```python
from build123d import *

# Parameters (mm, degrees)
EXTRUDE_1_DEPTH            = 7.5
EXTRUDE_1_DEPTH_BACK       = 7.5
SKETCH_3_W                 = 10
SKETCH_3_H                 = 21
CUT_EXTRUDE_1_DEPTH        = 29.062430401
SKETCH_4_W                 = 3
SKETCH_4_H                 = 3
EXTRUDE_2_DEPTH            = 1
EXTRUDE_3_DEPTH            = 2
EXTRUDE_3_DEPTH_BACK       = 2
CUT_EXTRUDE_2_REACH        = 27.53
SKETCH_7_W                 = 3
SKETCH_7_H                 = 3
EXTRUDE_4_DEPTH            = 1
EXTRUDE_START              = -4
EXTRUDE_5_DEPTH            = 5
CUT_EXTRUDE_3_REACH        = 28.373
SKETCH_10_R                = 1.9
EXTRUDE_6_DEPTH            = 1.5
EXTRUDE_START_2            = 1.5
SKETCH_11_R                = 1.9
EXTRUDE_7_DEPTH            = 1.5
EXTRUDE_8_DEPTH            = 0.5
EXTRUDE_8_DEPTH_BACK       = 0.5
SKETCH_13_W                = 12
SKETCH_13_H                = 1.5
EXTRUDE_9_DEPTH            = 1
CHAMFER_1_SIZE             = 1
CHAMFER_1_OF_MIRROR_2_SIZE = 1
FILLET_1_R                 = 0.1
FILLET_2_R                 = 0.2
FILLET_3_R                 = 0.2
FILLET_4_R                 = 0.1


with BuildPart() as part:
    # Sketch 1 → Extrude 1 (new, two sides: drawn at the far end of the back side and taken through both)
    with BuildSketch(Plane.XY.offset(-EXTRUDE_1_DEPTH_BACK)):
        with BuildLine():
            Line((-7.5, 0), (7.5, 0))
            Line((7.5, 0), (7.5, 15))
            ThreePointArc((7.5, 15), (0, 22.5), (-7.5, 15))
            Line((-7.5, 15), (-7.5, 0))
        make_face()
    extrude(amount=EXTRUDE_1_DEPTH + EXTRUDE_1_DEPTH_BACK)

    # Sketch 3 → Cut-Extrude 1 (cut, through all)
    with BuildSketch(Plane.ZY.offset(7.5)):
        with Locations((0, 12)):
            Rectangle(SKETCH_3_W, SKETCH_3_H)
    extrude(amount=-CUT_EXTRUDE_1_DEPTH, mode=Mode.SUBTRACT)

    # Sketch 4 → Extrude 2 (add)
    with BuildSketch(Plane(origin=(0, 0, 0), x_dir=(-1, 0, 0), z_dir=(0, -1, 0))):
        Rectangle(SKETCH_4_W, SKETCH_4_H)
    extrude(amount=EXTRUDE_2_DEPTH)

    # Sketch 5 → Extrude 3 (add, two sides: drawn at the far end of the back side and taken through both)
    with BuildSketch(Plane.XY.offset(-EXTRUDE_3_DEPTH_BACK)):
        with BuildLine():
            Line((-1.95, -2.5), (1.95, -2.5))
            Line((1.95, -2.5), (1.95, -1.555590279))
            ThreePointArc((1.95, -1.555590279), (1.780042303, -1.088161527), (1.5, -0.677124344))
            Line((1.5, -0.677124344), (-1.5, -0.677124344))
            ThreePointArc((-1.5, -0.677124344), (-1.780042303, -1.088161527), (-1.95, -1.555590279))
            Line((-1.95, -1.555590279), (-1.95, -2.5))
        make_face()
    extrude(amount=EXTRUDE_3_DEPTH + EXTRUDE_3_DEPTH_BACK)

    # Sketch 6 → Cut-Extrude 2 (cut, up to next)
    with BuildSketch(Plane.ZY.offset(1.95), mode=Mode.PRIVATE) as cut_extrude_2_sk1:
        with BuildLine():
            Line((-1.95, -2.5), (-1.95, -1.555590279))
            ThreePointArc((-1.95, -1.555590279), (-1.780042303, -1.088161527), (-1.5, -0.677124344))
            Line((-1.5, -0.677124344), (-2, -0.677124344))
            Line((-2, -0.677124344), (-2, -2.5))
            Line((-2, -2.5), (-1.95, -2.5))
        make_face()
    cut_extrude_2_tool1 = extrude(cut_extrude_2_sk1.sketch, amount=-CUT_EXTRUDE_2_REACH, mode=Mode.PRIVATE) & part.part
    # Sketch 6 → Cut-Extrude 2 (cut, up to next)
    with BuildSketch(Plane.ZY.offset(1.95), mode=Mode.PRIVATE) as cut_extrude_2_sk2:
        with BuildLine():
            Line((2, -2.5), (2, -0.677124344))
            Line((2, -0.677124344), (1.5, -0.677124344))
            ThreePointArc((1.5, -0.677124344), (1.780042303, -1.088161527), (1.95, -1.555590279))
            Line((1.95, -1.555590279), (1.95, -2.5))
            Line((1.95, -2.5), (2, -2.5))
        make_face()
    cut_extrude_2_tool2 = extrude(cut_extrude_2_sk2.sketch, amount=-CUT_EXTRUDE_2_REACH, mode=Mode.PRIVATE) & part.part
    add(cut_extrude_2_tool1.solids().sort_by_distance((-1.95, -1.175075, -1.873038))[0], mode=Mode.SUBTRACT)
    add(cut_extrude_2_tool2.solids().sort_by_distance((-1.95, -1.175075, 1.873038))[0], mode=Mode.SUBTRACT)

    # Sketch 7 → Extrude 4 (add)
    with BuildSketch(Plane.XY.offset(7.5)):
        with Locations((0, 15)):
            Rectangle(SKETCH_7_W, SKETCH_7_H)
    extrude_4 = extrude(amount=EXTRUDE_4_DEPTH)

    # Sketch 8 → Extrude 5 (add)
    with BuildSketch(Plane(origin=(0, 16.5, 0), x_dir=(1, 0, 0), z_dir=(0, 1, 0)).offset(EXTRUDE_START)):
        with BuildLine():
            Line((-1.95, -10), (1.95, -10))
            Line((1.95, -10), (1.95, -9.055590279))
            ThreePointArc((1.95, -9.055590279), (1.780042303, -8.588161527), (1.5, -8.177124344))
            Line((1.5, -8.177124344), (-1.5, -8.177124344))
            ThreePointArc((-1.5, -8.177124344), (-1.780042303, -8.588161527), (-1.95, -9.055590279))
            Line((-1.95, -9.055590279), (-1.95, -10))
        make_face()
    extrude_5 = extrude(amount=EXTRUDE_5_DEPTH)

    # Sketch 9 → Cut-Extrude 3 (cut, up to next)
    with BuildSketch(Plane.ZY.offset(1.95), mode=Mode.PRIVATE) as cut_extrude_3_sk1:
        with BuildLine():
            Line((10, 16.95), (9.055590279, 16.95))
            ThreePointArc((9.055590279, 16.95), (8.588161527, 16.780042303), (8.177124344, 16.5))
            Line((8.177124344, 16.5), (8.177124344, 17.5))
            Line((8.177124344, 17.5), (10, 17.5))
            Line((10, 17.5), (10, 16.95))
        make_face()
    cut_extrude_3_tool1 = extrude(cut_extrude_3_sk1.sketch, amount=-CUT_EXTRUDE_3_REACH, mode=Mode.PRIVATE) & part.part
    # Sketch 9 → Cut-Extrude 3 (cut, up to next)
    with BuildSketch(Plane.ZY.offset(1.95), mode=Mode.PRIVATE) as cut_extrude_3_sk2:
        with BuildLine():
            Line((10, 12.5), (8.177124344, 12.5))
            Line((8.177124344, 12.5), (8.177124344, 13.5))
            ThreePointArc((8.177124344, 13.5), (8.588161527, 13.219957697), (9.055590279, 13.05))
            Line((9.055590279, 13.05), (10, 13.05))
            Line((10, 13.05), (10, 12.5))
        make_face()
    cut_extrude_3_tool2 = extrude(cut_extrude_3_sk2.sketch, amount=-CUT_EXTRUDE_3_REACH, mode=Mode.PRIVATE) & part.part
    cut_extrude_3_1 = cut_extrude_3_tool1.solids().sort_by_distance((-1.95, 17.169375, 9.000125))[0]
    add(cut_extrude_3_1, mode=Mode.SUBTRACT)
    cut_extrude_3_2 = cut_extrude_3_tool2.solids().sort_by_distance((-1.95, 12.830625, 9.000125))[0]
    add(cut_extrude_3_2, mode=Mode.SUBTRACT)
    cut_extrude_3 = cut_extrude_3_1 + cut_extrude_3_2  # Cut-Extrude 3 as one shape, for the pattern or mirror that repeats it

    # Sketch 10 → Extrude 6 (add)
    with BuildSketch(Plane.XY.offset(-5)):
        with Locations(Location((0, 15, 0), (0, 0, 180))):
            Circle(SKETCH_10_R)
    extrude(amount=EXTRUDE_6_DEPTH)

    # Sketch 11 → Extrude 7 (add)
    with BuildSketch(Plane(origin=(0, 0, 5), x_dir=(-1, 0, 0), z_dir=(0, 0, -1)).offset(EXTRUDE_START_2)):
        with Locations((0, 15)):
            Circle(SKETCH_11_R)
    extrude(amount=-EXTRUDE_7_DEPTH)

    # Mirror 1: Extrude 4, Extrude 5, Cut-Extrude 3 across plane
    add(extrude_4.mirror(Plane.XY))
    add(extrude_5.mirror(Plane.XY))
    add(cut_extrude_3.mirror(Plane.XY), mode=Mode.SUBTRACT)

    # Sketch 12 → Extrude 8 (add, two sides: drawn at the far end of the back side and taken through both)
    with BuildSketch(Plane(origin=(0, 0, 0), x_dir=(0, 0, -1), z_dir=(1, 0, 0)).offset(-EXTRUDE_8_DEPTH_BACK)):
        Polygon((5, 1.5), (3, 1.5), (5, 3.5), align=None)
        Polygon((-5, 1.5), (-3, 1.5), (-5, 3.5), align=None)
    extrude(amount=EXTRUDE_8_DEPTH + EXTRUDE_8_DEPTH_BACK)

    # Sketch 13 → Extrude 9 (add)
    with BuildSketch(Plane.XY.offset(7.5)):
        with Locations((0, 6.75)):
            Rectangle(SKETCH_13_W, SKETCH_13_H)
    extrude_9 = extrude(amount=EXTRUDE_9_DEPTH)

    # Chamfer 1
    chamfer_1_edges = [part.edges().sort_by_distance(p)[0] for p in [
        (-6, 6.75, 8.5),
        (6, 6.75, 8.5),
    ]]
    chamfer(chamfer_1_edges, length=CHAMFER_1_SIZE - 0.0001)  # a hair under: the kernel refuses the full size

    # Mirror 2: Extrude 9 across plane
    add(extrude_9.mirror(Plane.XY))

    # Chamfer 1 of Mirror 2
    chamfer_1_of_mirror_2_edges = [part.edges().sort_by_distance(p)[0] for p in [
        (-6, 6.75, -8.5),
        (6, 6.75, -8.5),
    ]]
    chamfer(chamfer_1_of_mirror_2_edges, length=CHAMFER_1_OF_MIRROR_2_SIZE - 0.0001)  # a hair under: the kernel refuses the full size

    # Fillet 1
    fillet_1_edges = [part.edges().sort_by_distance(p)[0] for p in [
        (0, 16.95, 10),
        (-1.95, 15, 10),
        (1.95, 15, 10),
        (0, 13.05, 10),
        (0, 16.95, -10),
        (1.95, 15, -10),
        (-1.95, 15, -10),
        (0, 13.05, -10),
    ]]
    fillet(fillet_1_edges, radius=FILLET_1_R)

    # Fillet 2
    fillet_2_edges = [part.edges().sort_by_distance(p)[0] for p in [
        (7.5, 7.5, -7.5),
        (-7.5, 7.5, 7.5),
        (0, 0, 7.5),
        (0, 22.5, -7.5),
        (7.5, 7.5, 7.5),
        (0, 22.5, 7.5),
        (7.5, 8.25, -5),
        (0, 22.5, -5),
        (0, 22.5, 5),
        (7.5, 8.25, 5),
        (7.5, 1.5, 0),
        (-7.5, 8.25, 5),
        (-7.5, 8.25, -5),
        (-7.5, 1.5, 0),
        (-7.5, 7.5, -7.5),
        (0, 0, -7.5),
        (7.5, 0, 0),
        (-7.5, 0, 0),
    ]]
    fillet(fillet_2_edges, radius=FILLET_2_R)

    # Fillet 3
    fillet_3_edges = [part.edges().sort_by_distance(p)[0] for p in [
        (1.9, 15, -3.5),
        (1.9, 15, 3.5),
    ]]
    fillet(fillet_3_edges, radius=FILLET_3_R)

    # Fillet 4
    fillet_4_edges = [part.edges().sort_by_distance(p)[0] for p in [
        (1.95, -2.5, 0),
        (-1.95, -2.5, 0),
        (0, -2.5, -1.95),
        (0, -2.5, 1.95),
    ]]
    fillet(fillet_4_edges, radius=FILLET_4_R)


solid = part.part
```
Could you check a few things on this model? Use its own coordinates, in mm. A direction names the side the tool comes from. Coordinates: 2 decimals unless noted, no trailing zeros. Loops run counter-clockwise (first coordinate to the right, second up) from the corner with the lowest first, then second, coordinate; pieces in that order, holes last. Notation, with made-up numbers: M 14,-28.75 L 30,-28.75 A26 cw 30,-13.75 Z; hole C -35.75,27 d2. An arc over 180 degrees is marked long. Put each result on its own line as item: value. Start each with the question number.
(1) Suppose I cut it at D-D on z = -6.5. Please give me the cut outline in (x, y).
(2) Will these pins go through, and if not, where does the flat tip stop? P1, Ø1, axis at x = -2.5, y = 9, coming from the +Z side; P2, Ø0.9, axis at y = 14.5, z = 9.5, coming from the -X side; P3, Ø1, axis at y = 2.5, z = -3.5, coming from the +X side; P4, Ø0.6, axis at y = 3, z = 3.5, coming from the -X side.
(3) I need wall thicknesses on line 1 (Z direction, x = 3.5, y = 18); line 2 (Y direction, x = 2, z = 0.5); line 3 (Y direction, x = 2.25, z = -8). Which ranges of each line are inside material? Lowest first, please. Write a range as from..to.
(4) Suppose I cut it at A-A on y = 10.25. Please give me the cut outline in (x, z), then the cut area to 3 significant figures.
(5) For faces 1 (the face through (1.78, 14.97, -8.59)), 2 (the face through (-1.777, 14.973, -8.582)), 3 (the face through (0, 15, 3.5)), 4 (the face through (-1.021, 13.398, -4.359)), which set-ups out of +Z, -Z, +X, -X, +Y, -Y let a thin tool reach every point of the face, with its end or its side?
(6) Thinking about a two-plate mould opening in Z: for faces 5 (the face through (5.5, 6.7, -8)), 6 (the face through (0, 13.05, 9.5)), 7 (the face through (0, 15, -3.5)), which applies, pulls with the +Z half, pulls with the -Z half, needs draft (parallel to the pull), parting line crosses it, or undercut?
(7) Suppose I cut it at B-B on z = -0.25. Please give me the cut outline in (x, y), then the cut area to 3 significant figures.
Solutions:
1. outline: M -7.5,0.2 A0.2 ccw -7.3,0 L 7.3,0 A0.2 ccw 7.5,0.2 L 7.5,15 A7.5 ccw -7.5,15 Z
2. P1: stops at z = 7.5
2. P2: stops at x = -1.95
2. P3: stops at x = 0.5
2. P4: passes through
3. line 1: z = -7.5..-5, 5..7.5
3. line 2: y = 0..1.5
3. line 3: y = 6..7.5
4. outline: M -7.5,-7.3 A0.2 ccw -7.3,-7.5 L 7.3,-7.5 A0.2 ccw 7.5,-7.3 L 7.5,-5.2 A0.2 ccw 7.3,-5 L -7.3,-5 A0.2 ccw -7.5,-5.2 Z; M -7.5,5.2 A0.2 ccw -7.3,5 L 7.3,5 A0.2 ccw 7.5,5.2 L 7.5,7.3 A0.2 ccw 7.3,7.5 L -7.3,7.5 A0.2 ccw -7.5,7.3 Z
4. area: 74.9 mm2
5. face 1: +X, +Y
5. face 2: -X, +Y
5. face 3: +X, -X, +Y
5. face 4: none
6. face 5: pulls with the -Z half
6. face 6: needs draft
6. face 7: undercut
7. outline: M -7.5,0.2 A0.2 ccw -7.3,0 L -1.5,0 L -1.5,-0.68 A2 ccw -1.95,-1.56 L -1.95,-2.4 A0.1 ccw -1.85,-2.5 L 1.85,-2.5 A0.1 ccw 1.95,-2.4 L 1.95,-1.56 A2 ccw 1.5,-0.68 L 1.5,0 L 7.3,0 A0.2 ccw 7.5,0.2 L 7.5,1.3 A0.2 ccw 7.3,1.5 L -7.3,1.5 A0.2 ccw -7.5,1.3 Z
7. area: 31.3 mm2
